Can you work these out from the model? Positions are in its coordinate system, mm. A direction names the side the tool comes from. Give positions to 0.01 mm unless a question says otherwise; leave off trailing zeros. Write each loop counter-clockwise with the first axis right and the second up, starting at its lowest first coordinate (ties: lowest second). Pieces come first, ordered by that corner, then holes.
from build123d import *

# Parameters (mm, degrees)
SKETCH_1_W       = 214.117990109
SKETCH_1_H       = 65.359241046
EXTRUDE_1_DEPTH  = 3
SKETCH_2_R       = 2
EXTRUDE_2_DEPTH  = 12
SKETCH_3_R       = 2
EXTRUDE_3_DEPTH  = 12
SKETCH_4_R       = 2
EXTRUDE_4_DEPTH  = 12
SKETCH_5_R       = 3
EXTRUDE_5_DEPTH  = 8
SKETCH_6_R       = 4
EXTRUDE_6_DEPTH  = 1
SKETCH_7_R       = 3
EXTRUDE_7_DEPTH  = 8
SKETCH_8_R       = 3
EXTRUDE_8_DEPTH  = 8
SKETCH_9_R       = 4
EXTRUDE_9_DEPTH  = 1
SKETCH_10_R      = 4
EXTRUDE_10_DEPTH = 1


with BuildPart() as part:
    # 草图1 → 凸台-拉伸1 (new body)
    with BuildSketch(Plane(origin=(0, 0, 0), x_dir=(0, 0, -1), z_dir=(1, 0, 0))):
        with Locations((-107.058995055, 32.679620523)):
            Rectangle(SKETCH_1_W, SKETCH_1_H)
    extrude(amount=EXTRUDE_1_DEPTH)

    # 草图2 → 凸台-拉伸2 (add)
    with BuildSketch(Plane(origin=(3, 0, 0), x_dir=(0, 0, -1), z_dir=(1, 0, 0))):
        with Locations((-5.33476711, 57.554484424)):
            Circle(SKETCH_2_R)
    extrude(amount=EXTRUDE_2_DEPTH)

    # 草图3 → 凸台-拉伸3 (add)
    with BuildSketch(Plane(origin=(3, 0, 0), x_dir=(0, 0, -1), z_dir=(1, 0, 0))):
        with Locations((-105.33476711, 57.554484424)):
            Circle(SKETCH_3_R)
    extrude(amount=EXTRUDE_3_DEPTH)

    # 草图4 → 凸台-拉伸4 (add)
    with BuildSketch(Plane(origin=(3, 0, 0), x_dir=(0, 0, -1), z_dir=(1, 0, 0))):
        with Locations((-205.33476711, 57.554484424)):
            Circle(SKETCH_4_R)
    extrude(amount=EXTRUDE_4_DEPTH)

    # 草图5 → 凸台-拉伸5 (add)
    with BuildSketch(Plane(origin=(3, 0, 0), x_dir=(0, 0, -1), z_dir=(1, 0, 0))):
        with Locations((-5.33476711, 57.554484424)):
            Circle(SKETCH_5_R)
    extrude(amount=EXTRUDE_5_DEPTH)

    # 草图6 → 凸台-拉伸6 (add)
    with BuildSketch(Plane(origin=(3, 0, 0), x_dir=(0, 0, -1), z_dir=(1, 0, 0))):
        with Locations((-5.33476711, 57.554484424)):
            Circle(SKETCH_6_R)
    extrude(amount=EXTRUDE_6_DEPTH)

    # 草图7 → 凸台-拉伸7 (add)
    with BuildSketch(Plane(origin=(3, 0, 0), x_dir=(0, 0, -1), z_dir=(1, 0, 0))):
        with Locations((-105.33476711, 57.554484424)):
            Circle(SKETCH_7_R)
    extrude(amount=EXTRUDE_7_DEPTH)

    # 草图8 → 凸台-拉伸8 (add)
    with BuildSketch(Plane(origin=(3, 0, 0), x_dir=(0, 0, -1), z_dir=(1, 0, 0))):
        with Locations((-205.33476711, 57.554484424)):
            Circle(SKETCH_8_R)
    extrude(amount=EXTRUDE_8_DEPTH)

    # 草图9 → 凸台-拉伸9 (add)
    with BuildSketch(Plane(origin=(3, 0, 0), x_dir=(0, 0, -1), z_dir=(1, 0, 0))):
        with Locations((-105.33476711, 57.554484424)):
            Circle(SKETCH_9_R)
    extrude(amount=EXTRUDE_9_DEPTH)

    # 草图10 → 凸台-拉伸10 (add)
    with BuildSketch(Plane(origin=(3, 0, 0), x_dir=(0, 0, -1), z_dir=(1, 0, 0))):
        with Locations((-205.33476711, 57.554484424)):
            Circle(SKETCH_10_R)
    extrude(amount=EXTRUDE_10_DEPTH)


solid = part.part
(1) Imagine slicing it at A-A, the plane y = 30.5. Write out the boundary of the cut face in (x, z), plus the area to 3 significant figures.
Returned:
outline: (0, 0) - (3, 0) - (3, 214.12) - (0, 214.12) - close
area: 642 mm2
(2) Imagine slicing it at B-B, the plane z = 36.5. Write out the boundary of the cut face in (x, y), plus the area to 3 significant figures.
Returned:
outline: (0, 0) - (3, 0) - (3, 65.36) - (0, 65.36) - close
area: 196 mm2
(3) If we mould it in two halves opening along Z, with no side actions, what happens to faces 3 (the face through (0, 33, 109)), 4 (the face through (3.49, 57.73, 109.33))? For each: +Z half, -Z half, draft (parallel to the pull), parting line (faces both ways), or undercut.
Returned:
face 3: draft
face 4: undercut
(4) Imagine slicing it at C-C, the plane x = 6.75. Write out the boundary of the cut face in (y, z).
Returned:
outline: circle Ø6 at (57.55, 5.33); circle Ø6 at (57.55, 105.33); circle Ø6 at (57.55, 205.33)
(5) If I drill on L1, parallel to Z at x = 7.5, y = 57; L2, parallel to X at y = 16, z = 146; L3, parallel to Y at x = 6.75, z = 108, over which ranges is the centre line in solid material (lowest first)?
Returned:
L1: z = 2.39 to 8.28, 102.39 to 108.28, 202.39 to 208.28
L2: x = 0 to 3
L3: y = 56.18 to 58.93
(6) For faces 1 (the face through (12.972, 56.338, 206.922)), 2 (the face through (15, 58, 105)), which set-ups out of +Z, -Z, +X, -X, +Y, -Y let a thin tool reach every point of the face, with its end or its side?
Returned:
face 1: +X
face 2: +Z, -Z, +X, +Y, -Y
(7) Will these pins go through, and if not, where does the flat tip stop? P1, Ø10, axis at y = 11.5, z = 135, coming from the +X side; P2, Ø1.5, axis at x = 3.5, y = 44, coming from the -Z side.
Returned:
P1: stops at x = 3
P2: stops at z = 0
